Input: part model. Units: mm. Frame: model coordinates. Face numbers are marked on the shaded views. A direction names the side the tool comes from. Round coordinates to 2 decimals unless told otherwise and drop trailing zeros. Loops run counter-clockwise (first coordinate to the right, second up) from the corner with the lowest first, then second, coordinate; pieces in that order, holes last. Notation, with made-up numbers: M 76.25,9 L 96.25,9 A27 cw 96.25,47 Z; hole C 75.25,36 d6. An arc over 180 degrees is marked long. Use one line per item in the form item = value. Start each with the question number.
Q1. Access query for the marked faces 1 and 2. Directions: +Z, -Z, +X, -X, +Y, -Y. A direction counts if a zero-diameter tool reaches every point of the face in a straight line with its end or side. Return the directions, or none.
Q2. Mould query, pull axis Y, two halves, no side actions, for the marked faces 3, 4 and 5. Classes: pulls with the +Y half, pulls with the -Y half, needs draft (parallel to the pull), parting line crosses it, or undercut.
Q3. Ray query, line 1 along Y through (x, z) = (-20, 3.95); line 2 along Y through (x, z) = (-0.5, 9.25); line 3 along Y through (x, z) = (0, 1.05) (3 decimals). Return the intervals inside material, ascending.
Q4. First-contact query: P1, Ø2, axis at x = 16, y = 1.5, coming from the +Z side; P2, Ø1.5, axis at y = 9.5, z = 7, coming from the -X side; P3, Ø2, axis at x = -11.5, z = 8.5, coming from the +Y side. Flat tips, straight axial feed; report the tip coordinate or a pass-through.
Q5. Section query A-A, the plane z = 10.5. Output: boundary loops of the cut face in (x, y).
```python
from build123d import *

# Parameters (mm, degrees)
ESQUISSE1_W             = 50
ESQUISSE1_H             = 50
BOSS_EXTRU_3_DEPTH      = 5
ESQUISSE3_R             = 22.5
ESQUISSE3_R_2           = 20.5
BOSS_EXTRU_4_DEPTH      = 8
ENL_V_MAT_EXTRU_1_DEPTH = 2
ESQUISSE5_R             = 0.65
ESQUISSE5_R_2           = 1.375
ENL_V_MAT_EXTRU_2_DEPTH = 37.742346142
CONG_1_R                = 5
ESQUISSE6_R             = 1.5
ENL_V_MAT_EXTRU_3_DEPTH = 37.249137921
CONG_2_R                = 1
CONG_3_R                = 1


with BuildPart() as part:
    # Esquisse1 → Boss.-Extru.3 (new body)
    with BuildSketch(Plane.XY):
        Rectangle(ESQUISSE1_W, ESQUISSE1_H)
    extrude(amount=BOSS_EXTRU_3_DEPTH)

    # Esquisse3 → Boss.-Extru.4 (add)
    with BuildSketch(Plane.XY.offset(5)):
        Circle(ESQUISSE3_R)
        Circle(ESQUISSE3_R_2, mode=Mode.SUBTRACT)
    extrude(amount=BOSS_EXTRU_4_DEPTH)

    # Esquisse4 → Enlèv. mat.-Extru.1 (cut)
    with BuildSketch(Plane.XY.offset(5)):
        with BuildLine():
            Line((-14.148131749, 1.273093878), (-2.594747862, 2.266121915))
            ThreePointArc((-2.594747862, 2.266121915), (-0.147642857, 3.44183477), (2.391155578, 2.48))
            Line((2.391155578, 2.48), (13.987136948, 2.48))
            ThreePointArc((13.987136948, 2.48), (15.866074919, 0.663183078), (14.113431719, -1.275753084))
            Line((14.113431719, -1.275753084), (2.594747862, -2.266121915))
            ThreePointArc((2.594747862, -2.266121915), (0.147642857, -3.44183477), (-2.391155578, -2.48))
            Line((-2.391155578, -2.48), (-13.987136948, -2.48))
            ThreePointArc((-13.987136948, -2.48), (-15.865409624, -0.680571429), (-14.148131749, 1.273093878))
        make_face()
    extrude(amount=-ENL_V_MAT_EXTRU_1_DEPTH, mode=Mode.SUBTRACT)

    # Esquisse5 → Enlèv. mat.-Extru.2 (cut, through all)
    with BuildSketch(Plane.XY.offset(3)):
        with Locations((-14.236907251, -0.610714286)):
            Circle(ESQUISSE5_R)
        with Locations((14.236907251, 0.610714286)):
            Circle(ESQUISSE5_R)
        Circle(ESQUISSE5_R_2)
    extrude(amount=-ENL_V_MAT_EXTRU_2_DEPTH, mode=Mode.SUBTRACT)

    # Congé1
    cong_1_edges = [part.edges().sort_by_distance(p)[0] for p in [
        (25, -25, 2.5),
        (-25, -25, 2.5),
        (-25, 25, 2.5),
        (25, 25, 2.5),
    ]]
    fillet(cong_1_edges, radius=CONG_1_R)

    # Esquisse6 → Enlèv. mat.-Extru.3 (cut, through all)
    with BuildSketch(Plane.XY.offset(5)):
        with Locations((-20, -20)):
            Circle(ESQUISSE6_R)
        with Locations((20, -20)):
            Circle(ESQUISSE6_R)
        with Locations((20, 20)):
            Circle(ESQUISSE6_R)
        with Locations((-20, 20)):
            Circle(ESQUISSE6_R)
    extrude(amount=-ENL_V_MAT_EXTRU_3_DEPTH, mode=Mode.SUBTRACT)

    # Congé2
    cong_2_edges = [part.edges().sort_by_distance(p)[0] for p in [
        (-22.5, 0, 5),
    ]]
    fillet(cong_2_edges, radius=CONG_2_R)

    # Congé3
    cong_3_edges = [part.edges().sort_by_distance(p)[0] for p in [
        (-22.5, 0, 13),
    ]]
    fillet(cong_3_edges, radius=CONG_3_R)


solid = part.part
```
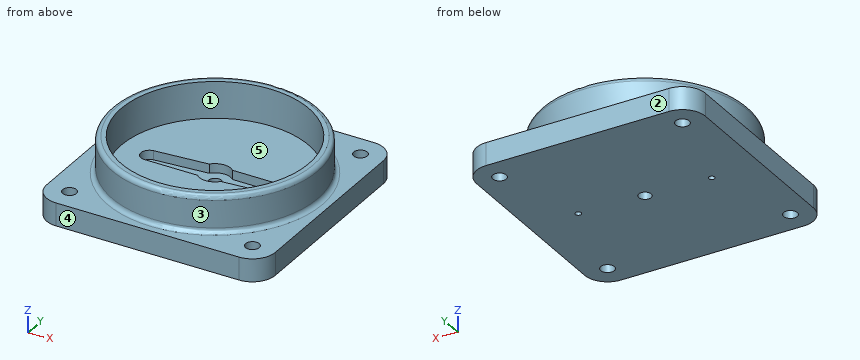
Results found:
q1.face_1 = +Z
q1.face_2 = +Z, -Z, +X, -X, +Y
q2.face_3 = parting line crosses it
q2.face_4 = pulls with the -Y half
q2.face_5 = undercut
q3.line_1 = -25 to -21.5, -18.5 to 18.5, 21.5 to 25
q3.line_2 = -22.49 to -20.49, 20.49 to 22.49
q3.line_3 = -25 to -1.375, 1.375 to 25
q4.P1 = 5
q4.P2 = -20.73
q4.P3 = 19.9
q5.outline = C 0,0 d45; hole C 0,0 d41
